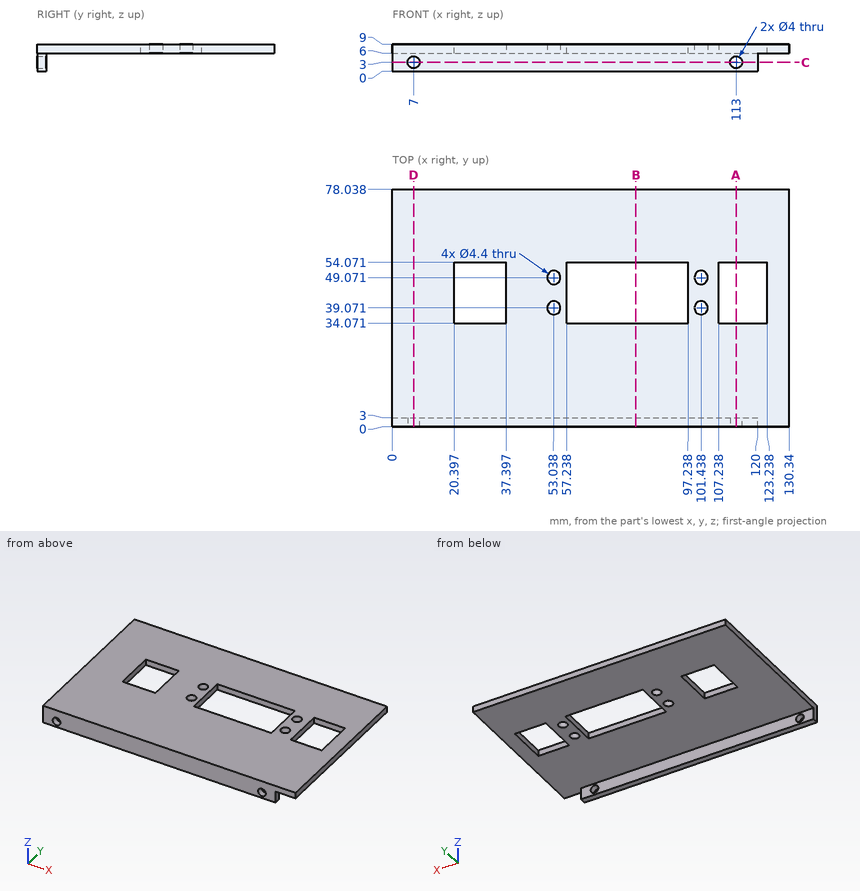
The drawing under review shows one solid part. Ordinate dimensions are in mm from its lowest x, y, z. Round coordinates to 2 decimals unless told otherwise and drop trailing zeros. Write each loop counter-clockwise with the first axis right and the second up, starting at its lowest first coordinate (ties: lowest second). Pieces come first, ordered by that corner, then holes.
(1) Wall thickness on L1, parallel to X at y = 52, z = 6.25; L2, parallel to Z at x = 7, y = 1; L3, parallel to Y at x = 85.5, z = 6.5: over which ranges is each line inside the solid? List them lowest first.
(2) We need section C-C on z = 3. Give the boundary of the cut face in (x, y).
(3) We need section A-A on x = 113. Give the boundary of the cut face in (y, z).
(4) We need section D-D on x = 7. Give the boundary of the cut face in (y, z).
(5) Insertion check: pin 1 (1.5 mm diameter, centred on x = 57, y = 48.5, fed in from -Z); pin 2 (2.5 mm diameter, centred on x = 53.04, y = 39.07, fed in from +Z); pin 3 (3.5 mm diameter, centred on y = 2, z = 2.5, fed in from +X). Each pin has a flat end and moves straight along its axis. Give the tip position at first contact, or say it passes through.
(6) We need section B-B on x = 80. Give the boundary of the cut face in (y, z), and give its area (3 significant figures).
Findings below:
1. L1: x = 0 to 20.4, 37.4 to 57.24, 97.24 to 107.24, 123.24 to 130.34
1. L2: z = 0 to 1, 5 to 9
1. L3: y = 0 to 34.07, 54.07 to 78.04
2. outline: (0, 0) - (5, 0) - (5, 3) - (0, 3) - close; (9, 0) - (111, 0) - (111, 3) - (9, 3) - close; (115, 0) - (120, 0) - (120, 3) - (115, 3) - close
3. outline: (0, 0) - (3, 0) - (3, 1) - (0, 1) - close; (0, 5) - (3, 5) - (3, 6) - (34.07, 6) - (34.07, 9) - (0, 9) - close; (54.07, 6) - (78.04, 6) - (78.04, 9) - (54.07, 9) - close
4. outline: (0, 0) - (3, 0) - (3, 1) - (0, 1) - close; (0, 5) - (3, 5) - (3, 6) - (78.04, 6) - (78.04, 9) - (0, 9) - close
5. pin 1: stops at z = 6
5. pin 2: passes through
5. pin 3: stops at x = 120
6. outline: (0, 0) - (3, 0) - (3, 6) - (34.07, 6) - (34.07, 9) - (0, 9) - close; (54.07, 6) - (78.04, 6) - (78.04, 9) - (54.07, 9) - close
6. area: 192 mm2
